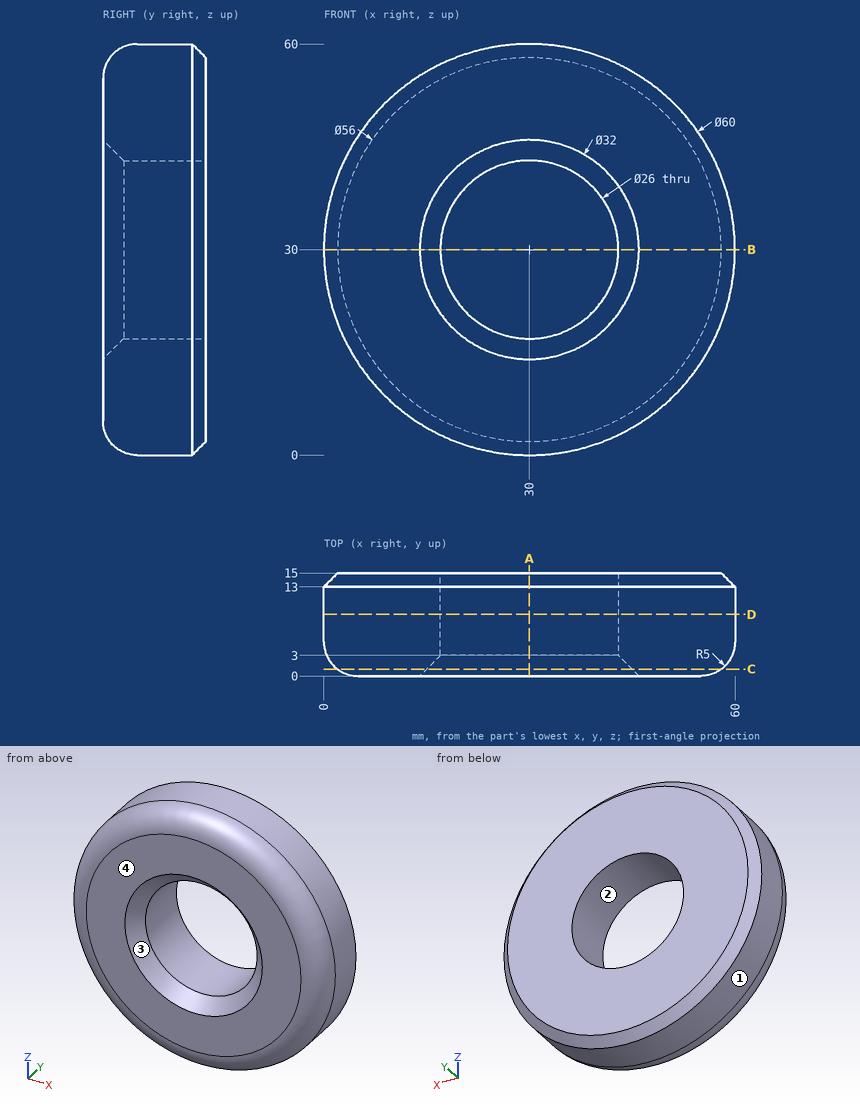
Verification items for this drawing (mm, ordinates from the low corner). Give positions to 0.01 mm unless a question says otherwise; leave off trailing zeros. Write each loop counter-clockwise with the first axis right and the second up, starting at its lowest first coordinate (ties: lowest second). Pieces come first, ordered by that corner, then holes. Notation, with made-up numbers: M 88.25,-36.75 L 96.25,-36.75 A27 cw 96.25,-12.75 Z; hole C 29,35 d5. An arc over 180 degrees is marked long. Use one line per item in the form item = value.
(1) Section check B-B on z = 30. Record the boundary of the cut face in (x, y), plus the area to 3 significant figures.
Answer block:
outline = M 0,5 A5 ccw 5,0 L 14,0 L 17,3 L 17,15 L 2,15 L 0,13 Z; M 43,3 L 46,0 L 55,0 A5 ccw 60,5 L 60,13 L 58,15 L 43,15 Z
area = 486 mm2
(2) Section check C-C on y = 1. Record the boundary of the cut face in (x, z).
Answer block:
outline = C 30,30 d56; hole C 30,30 d30
(3) Section check A-A on x = 30. Record the boundary of the cut face in (y, z).
Answer block:
outline = M 0,5 A5 ccw 5,0 L 13,0 L 15,2 L 15,17 L 3,17 L 0,14 Z; M 0,46 L 3,43 L 15,43 L 15,58 L 13,60 L 5,60 A5 ccw 0,55 Z
(4) Draft check along Z on the marked faces 1, 2, 3 and 4. Enter one of: pulls with the +Z half, pulls with the -Z half, needs draft (parallel to the pull), parting line crosses it, or undercut.
Answer block:
face_1 = parting line crosses it
face_2 = undercut
face_3 = undercut
face_4 = needs draft
(5) Section check D-D on y = 9. Record the boundary of the cut face in (x, z).
Answer block:
outline = C 30,30 d60; hole C 30,30 d26
(6) Material ranges on line 1 along Z through (x, y) = (30, 5.5); line 2 along X through (y, z) = (10, 29.5); line 3 along X through (y, z) = (5, 40), recorded low to high.
Answer block:
line_1 = 0 to 17, 43 to 60
line_2 = 0 to 17.01, 42.99 to 60
line_3 = 1.72 to 21.69, 38.31 to 58.28
(7) Depth check by flat-ended pin: P1, Ø3, axis at x = 52.5, y = 11.5, coming from the -Z side; P2, Ø4, axis at y = 6, z = 14.5, coming from the -X side; P3, Ø2, axis at x = 7.5, y = 7, coming from the +Z side; P4, Ø23.5, axis at x = 30, z = 30, coming from the -Y side. Enter the tip coordinate at first touch or a pass-through.
Answer block:
P1 = 8.58
P2 = 3.21
P3 = 50.92
P4 = through
